from build123d import *

# Parameters (mm, degrees)
SKETCH1_W                        = 88.9
SKETCH1_H                        = 533.4
BOSS_EXTRUDE1_DEPTH              = 38.1
F_3_8_0_375_DIAMETER_HOLE1_D     = 9.525
F_3_8_0_375_DIAMETER_HOLE1_DEPTH = 76.2
F_3_8_0_375_DIAMETER_HOLE1_TIP   = 2.861598698
SKETCH4_R                        = 4.7625
CUT_EXTRUDE1_DEPTH               = 543.098127648
SKETCH5_R                        = 4.7625
CUT_EXTRUDE2_DEPTH               = 543.098127648


with BuildPart() as part:
    # Sketch1 → Boss-Extrude1 (new body)
    with BuildSketch(Plane.XY):
        with Locations((44.45, 266.7)):
            Rectangle(SKETCH1_W, SKETCH1_H)
    extrude(amount=BOSS_EXTRUDE1_DEPTH)

    # 3/8 (0.375) Diameter Hole1
    with Locations(Plane.XY.offset(38.1)):
        with Locations((44.45, 488.95)):
            Hole(F_3_8_0_375_DIAMETER_HOLE1_D / 2, depth=F_3_8_0_375_DIAMETER_HOLE1_DEPTH)
            with Locations((0, 0, -(F_3_8_0_375_DIAMETER_HOLE1_DEPTH + F_3_8_0_375_DIAMETER_HOLE1_TIP / 2))):  # 118° drill point
                Cone(0, F_3_8_0_375_DIAMETER_HOLE1_D / 2, F_3_8_0_375_DIAMETER_HOLE1_TIP, mode=Mode.SUBTRACT)

    # Sketch4 → Cut-Extrude1 (cut, through all)
    with BuildSketch(Plane.XY.offset(38.1)):
        with Locations((44.45, 133.35)):
            Circle(SKETCH4_R)
    extrude(amount=-CUT_EXTRUDE1_DEPTH, mode=Mode.SUBTRACT)

    # Sketch5 → Cut-Extrude2 (cut, through all)
    with BuildSketch(Plane.XY.offset(38.1)):
        with Locations((44.45, 171.45)):
            Circle(SKETCH5_R)
    extrude(amount=-CUT_EXTRUDE2_DEPTH, mode=Mode.SUBTRACT)


solid = part.part
Work out the finished part from the listing and answer in its coordinate system (mm). Round coordinates to 2 decimals unless told otherwise and drop trailing zeros. Loops run counter-clockwise (first coordinate to the right, second up) from the corner with the lowest first, then second, coordinate; pieces in that order, holes last. Notation, with made-up numbers: (-3, 87) - (25, 87) arc R31 ccw to (25, 120) - close; hole circle Ø8 at (-7, -4). An arc over 180 degrees is marked (long way). One line per item, written item: value.
Q1. Find section B-B on x = 44.45. Give the vertices of the cut face in (y, z), and give its area (3 significant figures).
Check values:
outline: (0, 0) - (128.59, 0) - (128.59, 38.1) - (0, 38.1) - close; (138.11, 0) - (166.69, 0) - (166.69, 38.1) - (138.11, 38.1) - close; (176.21, 0) - (484.19, 0) - (484.19, 38.1) - (176.21, 38.1) - close; (493.71, 0) - (533.4, 0) - (533.4, 38.1) - (493.71, 38.1) - close
area: 19,200 mm2
Q2. Find section A-A on y = 488.95. Give the vertices of the cut face in (x, z), and give its area (3 significant figures).
Check values:
outline: (0, 0) - (39.69, 0) - (39.69, 38.1) - (0, 38.1) - close; (49.21, 0) - (88.9, 0) - (88.9, 38.1) - (49.21, 38.1) - close
area: 3,020 mm2
Q3. The mould has two halves that part along X. Classify faces 1 (the flat face through (0, 263, 19)), 2 (the flat face through (44, 270, 0)), 3 (the cylindrical face through (43.83, 176.17, 19.32)): +X half, -X half, draft (parallel to the pull), parting line (faces both ways), or undercut.
Check values:
face 1: -X half
face 2: draft
face 3: undercut
Q4. Straight lines are drawn through the part: probe 1 along Y at (x, z) = (44, 29); probe 2 along X at (y, z) = (171, 24); probe 3 along X at (y, z) = (488, 9). For each, find the intervals that lie inside material, in ascending order.
Check values:
probe 1: 0 to 128.61, 138.09 to 166.71, 176.19 to 484.21, 493.69 to 533.4
probe 2: 0 to 39.71, 49.19 to 88.9
probe 3: 0 to 39.78, 49.12 to 88.9
